The model under review builds one solid part; all positions refer to its coordinate system, in mm. Round coordinates to 2 decimals unless told otherwise and drop trailing zeros. Write each loop counter-clockwise with the first axis right and the second up, starting at its lowest first coordinate (ties: lowest second). Pieces come first, ordered by that corner, then holes.
Item 1: Add section C-C (x = 0). Give the boundary of the cut face in (y, z) (3 decimals).
Item 2: To check wall thickness, follow L1, parallel to X at y = 197.5, z = 2.05; L2, parallel to X at y = 302.5, z = 1.05; L3, parallel to Y at x = -6, z = 1.45. State the ranges of each line that lie inside material, in increasing order.
Item 3: Add section B-B (z = 1.95). Give the boundary of the cut face in (x, y), plus the area to 3 significant figures.
Item 4: Add section A-A (y = 277). Give the boundary of the cut face in (x, z) (3 decimals).
```python
from build123d import *

# Parameters (mm, degrees)
BOSS_EXTRUDE1_DEPTH = 3.175
CUT_EXTRUDE1_DEPTH  = 3.175


with BuildPart() as part:
    # Sketch1 → Boss-Extrude1 (new body)
    with BuildSketch(Plane.XY):
        with BuildLine():
            Line((175, 300), (175, 50))
            Line((175, 50), (125, 0))
            Line((125, 0), (50, 0))
            ThreePointArc((50, 0), (0, 50), (-50, 0))
            Line((-50, 0), (-125, 0))
            Line((-125, 0), (-175, 50))
            Line((-175, 50), (-175, 300))
            Line((-175, 300), (-125, 350))
            Line((-125, 350), (-50, 350))
            ThreePointArc((-50, 350), (0, 300), (50, 350))
            Line((50, 350), (125, 350))
            Line((125, 350), (175, 300))
        make_face()
    extrude(amount=BOSS_EXTRUDE1_DEPTH)

    # Sketch2 → Cut-Extrude1 (cut)
    with BuildSketch(Plane.XY.offset(3.175)):
        with BuildLine():
            Line((-25, 306.698729811), (-25, 150))
            ThreePointArc((-25, 150), (0, 125), (25, 150))
            Line((25, 150), (25, 306.698729811))
            ThreePointArc((25, 306.698729811), (0, 300), (-25, 306.698729811))
        make_face()
    extrude(amount=-CUT_EXTRUDE1_DEPTH, mode=Mode.SUBTRACT)


solid = part.part
```
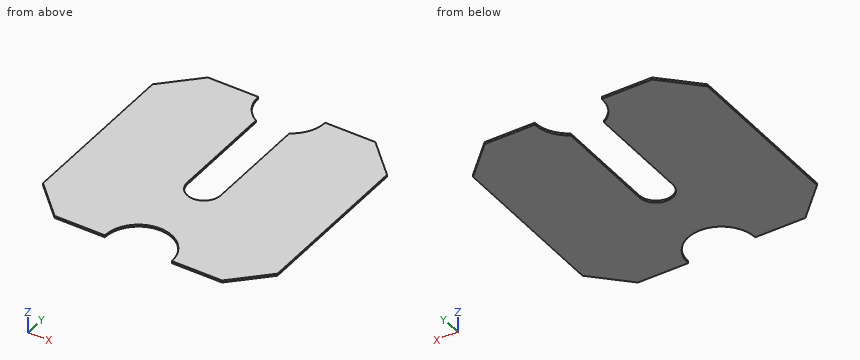
Numbers:
1. outline: (50, 0) - (125, 0) - (125, 3.175) - (50, 3.175) - close
2. L1: x = -175 to -25, 25 to 175
2. L2: x = -172.5 to -25, 25 to 172.5
2. L3: y = 49.64 to 125.73
3. outline: (-175, 50) - (-125, 0) - (-50, 0) arc R50 cw to (50, 0) - (125, 0) - (175, 50) - (175, 300) - (125, 350) - (50, 350) arc R50 cw to (25, 306.7) - (25, 150) arc R25 cw to (-25, 150) - (-25, 306.7) arc R50 cw to (-50, 350) - (-125, 350) - (-175, 300) - close
3. area: 101,000 mm2
4. outline: (-175, 0) - (-25, 0) - (-25, 3.175) - (-175, 3.175) - close; (25, 0) - (175, 0) - (175, 3.175) - (25, 3.175) - close
